Check sheet for the modelled part. Datum: model origin and axes. Units: mm. Face numbers are marked on the shaded views. Round coordinates to 2 decimals unless told otherwise and drop trailing zeros. Loops run counter-clockwise (first coordinate to the right, second up) from the corner with the lowest first, then second, coordinate; pieces in that order, holes last. Notation, with made-up numbers: (-31.5, 82.5) -> (23.5, 82.5) arc R27 ccw to (23.5, 103.5) -> close; hole circle Ø10 at (62, -20). An arc over 180 degrees is marked (long way). One line per item, written item: value. Start each with the question number.
1. Cross-section at A-A on y = 0. Record the cut outline in (x, z).
2. Material ranges on L1, parallel to Y at x = -0.05, z = 5.25; L2, parallel to Y at x = 1, z = 5.25; L3, parallel to Z at x = 1.6, y = -1.1, recorded low to high.
3. Release check for a two-part mould opening along Z. For the marked faces 1, 2 and 3 record: +Z half, -Z half, draft (parallel to the pull), parting line (faces both ways), or undercut.
4. Cross-section at C-C on z = 2. Record the cut outline in (x, y), then the cut area to 3 significant figures.
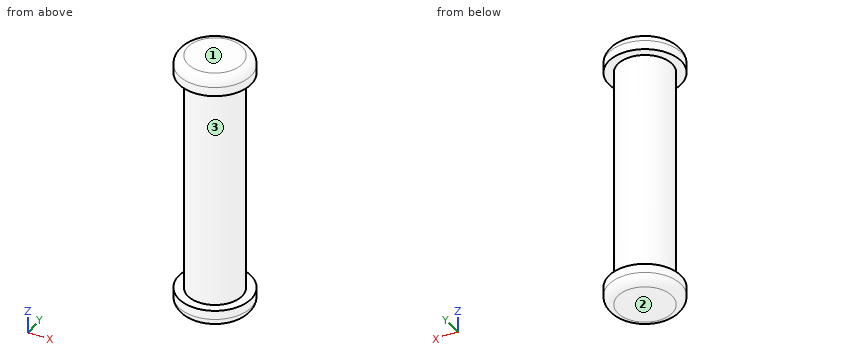
from build123d import *

# Parameters (mm, degrees)
SKETCH1_R           = 1.5
BOSS_EXTRUDE1_DEPTH = 12.5
SKETCH2_R           = 2
BOSS_EXTRUDE2_DEPTH = 1
SKETCH3_R           = 2
BOSS_EXTRUDE3_DEPTH = 1
FILLET1_R           = 0.5


with BuildPart() as part:
    # Sketch1 → Boss-Extrude1 (new body)
    with BuildSketch(Plane.XY):
        Circle(SKETCH1_R)
    extrude(amount=BOSS_EXTRUDE1_DEPTH)

    # Sketch2 → Boss-Extrude2 (add)
    with BuildSketch(Plane(origin=(0, 0, 0), x_dir=(-1, 0, 0), z_dir=(0, 0, -1))):
        Circle(SKETCH2_R)
    extrude(amount=BOSS_EXTRUDE2_DEPTH)

    # Sketch3 → Boss-Extrude3 (add)
    with BuildSketch(Plane.XY.offset(12.5)):
        Circle(SKETCH3_R)
    extrude(amount=BOSS_EXTRUDE3_DEPTH)

    # Fillet1
    fillet1_edges = [part.edges().sort_by_distance(p)[0] for p in [
        (-2, 0, 13.5),
        (2, 0, -1),
    ]]
    fillet(fillet1_edges, radius=FILLET1_R)


solid = part.part
Taken from the geometry:
1. outline: (-2, -0.5) arc R0.5 ccw to (-1.5, -1) -> (1.5, -1) arc R0.5 ccw to (2, -0.5) -> (2, 0) -> (1.5, 0) -> (1.5, 12.5) -> (2, 12.5) -> (2, 13) arc R0.5 ccw to (1.5, 13.5) -> (-1.5, 13.5) arc R0.5 ccw to (-2, 13) -> (-2, 12.5) -> (-1.5, 12.5) -> (-1.5, 0) -> (-2, 0) -> close
2. L1: y = -1.5 to 1.5
2. L2: y = -1.12 to 1.12
2. L3: z = -0.73 to 0, 12.5 to 13.23
3. face 1: +Z half
3. face 2: -Z half
3. face 3: undercut
4. outline: circle Ø3 at (0, 0)
4. area: 7.07 mm2
